Autodesk Inventor part; units mm, degrees
ref_plane "YZ Plane" through (0, 0, 0) normal (1, 0, 0) x (0, 1, 0)
ref_plane "XZ Plane" through (0, 0, 0) normal (0, 1, 0) x (-1, 0, 0)
ref_plane "XY Plane" through (0, 0, 0) normal (0, 0, 1) x (1, 0, 0)
sketch "Эскиз1" plane through (0, 0, 0) normal (0, 1, 0) x (-1, 0, 0)
  line L0 (0, 0) -> (70, 0)
  line L1 (70, 0) -> (70, -90)
  line L2 (70, -90) -> (0, -90)
  line L3 (0, -90) -> (0, 0)
  dimension "d0" = 70
  dimension "d1" = 90
extrude "Выдавливание1" add sketch "Эскиз1" along normal blind 1.5
sketch "Эскиз2" plane through (0, 1.5, 0) normal (0, 1, 0) x (1, 0, 0)
  line L0 (0, 0) -> (0, 90)
  line L1 (0, 0) -> (-7, 0)
  line L2 (-7, 0) -> (-7, 7)
  line L3 (-7, 7) -> (0, 7)
  line L4 (0, 7) -> (0, 0)
  line L5 (-70, 0) -> (0, 0)
  line L6 (-70, 0) -> (-63, 0)
  line L7 (-63, 0) -> (-63, 7)
  line L8 (-63, 7) -> (-70, 7)
  line L9 (-70, 7) -> (-70, 0)
  line L10 (0, 90) -> (-70, 90)
  line L11 (-70, 90) -> (-63, 90)
  line L12 (-63, 90) -> (-63, 83)
  line L13 (-63, 83) -> (-70, 83)
  line L14 (-70, 83) -> (-70, 90)
  line L15 (0, 90) -> (-7, 90)
  line L16 (-7, 90) -> (-7, 83)
  line L17 (-7, 83) -> (0, 83)
  line L18 (0, 83) -> (0, 90)
  point P0 (0, 7)
  point P1 (0, 83)
  point P2 (-63, 0)
  dimension "d4" = 7
  dimension "d5" = 7
  dimension "d6" = 7
  dimension "d7" = 7
  dimension "d8" = 7
  dimension "d9" = 7
  dimension "d10" = 7
  dimension "d11" = 7
extrude "Выдавливание2" add sketch "Эскиз2" along normal blind 5
sketch "Эскиз3" plane through (0, 6.5, 0) normal (0, 1, 0) x (1, 0, 0)
  circle A0 centre (-2.75, 86.25) radius 1.25
  circle A1 centre (-66.25, 86.25) radius 1.25
  circle A2 centre (-66.25, 3.75) radius 1.25
  circle A3 centre (-2.75, 3.75) radius 1.25
  line L0 (-63, 90) -> (-70, 90)
  line L1 (0, 90) -> (-7, 90)
  line L2 (-70, 0) -> (-63, 0)
  line L3 (-7, 0) -> (0, 0)
  line L4 (-70, 90) -> (-70, 83)
  line L5 (0, 7) -> (0, 83)
  line L6 (-70, 7) -> (-70, 0)
  line L7 (0, 0) -> (0, 7)
  dimension "d14" = 2.5
  dimension "d15" = 2.5
  dimension "d16" = 2.5
  dimension "d17" = 2.5
  dimension "d18" = 3.75
  dimension "d19" = 3.75
  dimension "d20" = 3.75
  dimension "d21" = 3.75
  dimension "d22" = 3.75
  dimension "d23" = 2.75
  dimension "d24" = 3.75
  dimension "d25" = 2.75
extrude "Выдавливание3" cut sketch "Эскиз3" against normal blind 5
fillet "Сопряжение1" radius 2 4 edges at (0, 3.25, 0) (0, 3.25, -90) (-70, 3.25, -90) (-70, 3.25, 0)
properties part number "SensorsC_Holder"
Source: CAD feature listing. Evaluate the final solid. Frame: model axes, mm. A direction names the side the tool comes from. Coordinates: 2 decimals unless noted, no trailing zeros. Loops run counter-clockwise (first coordinate to the right, second up) from the corner with the lowest first, then second, coordinate; pieces in that order, holes last. Notation, with made-up numbers: (49, 7) - (98, 7) arc R25 ccw to (98, 34) - close; hole circle Ø9 at (74.5, 50). An arc over 180 degrees is marked (long way). Answer as CSV lines item,"result".
1. Section A-A (y = 4.75). Return loops of the section in (x, z).
Established:
outline,"(-70, -88) arc R2 ccw to (-68, -90) - (-63, -90) - (-63, -83) - (-70, -83) - close; (-70, -7) - (-63, -7) - (-63, 0) - (-68, 0) arc R2 ccw to (-70, -2) - close; (-7, -90) - (-2, -90) arc R2 ccw to (0, -88) - (0, -83) - (-7, -83) - close; (-7, -7) - (0, -7) - (0, -2) arc R2 ccw to (-2, 0) - (-7, 0) - close; hole circle Ø2.5 at (-66.25, -86.25); hole circle Ø2.5 at (-66.25, -3.75); hole circle Ø2.5 at (-2.75, -86.25); hole circle Ø2.5 at (-2.75, -3.75)"
2. Contact query for flat-ended pins moving along their axis: pin 1 (1.5 mm diameter, centred on x = -38, z = -26, fed in from +Y); pin 2 (1.5 mm diameter, centred on x = -10.5, y = 3.5, fed in from +Z). Output: stop coordinate, or through.
Established:
pin 1,"stops at y = 1.5"
pin 2,"passes through"
3. Mould query, pull axis Z, two halves, no side actions, for faces 1 (the cylindrical face through (-65.095, 4.035, -3.271)), 2 (the cylindrical face through (-69.43, 3.2, -89.4)), 3 (the cylindrical face through (-0.6, 3.3, -0.57)), 4 (the flat face through (-7, 4, -3)). Classes: released by +Z, released by -Z, zero draft, split by the parting line, or undercut.
Established:
face 1,"undercut"
face 2,"released by -Z"
face 3,"released by +Z"
face 4,"zero draft"
4. Section C-C (z = -86.25). Return loops of the section in (x, y), then the cut area to 3 significant figures.
Established:
outline,"(-70, 0) - (0, 0) - (0, 6.5) - (-1.5, 6.5) - (-1.5, 1.5) - (-4, 1.5) - (-4, 6.5) - (-7, 6.5) - (-7, 1.5) - (-63, 1.5) - (-63, 6.5) - (-65, 6.5) - (-65, 1.5) - (-67.5, 1.5) - (-67.5, 6.5) - (-70, 6.5) - close"
area,"150 mm2"
5. Section B-B (x = -66.25). Return loops of the section in (y, z).
Established:
outline,"(0, -90) - (6.5, -90) - (6.5, -87.5) - (1.5, -87.5) - (1.5, -85) - (6.5, -85) - (6.5, -83) - (1.5, -83) - (1.5, -7) - (6.5, -7) - (6.5, -5) - (1.5, -5) - (1.5, -2.5) - (6.5, -2.5) - (6.5, 0) - (0, 0) - close"
6. Ray query, line 1 (X direction, y = 5.2, z = -3.75); line 2 (Z direction, x = -66.25, y = 3.3); line 3 (Z direction, x = -64, y = 4). Return the intervals inside material, ascending.
Established:
line 1,"x = -70 to -67.5, -65 to -63, -7 to -4, -1.5 to 0"
line 2,"z = -90 to -87.5, -85 to -83, -7 to -5, -2.5 to 0"
line 3,"z = -90 to -83, -7 to 0"
7. Section D-D (x = -46). Return loops of the section in (y, z).
Established:
outline,"(0, -90) - (1.5, -90) - (1.5, 0) - (0, 0) - close"
8. Reachability of faces 5 (the flat face through (-66, 4, -83)), 6 (the cylindrical face through (-2.173, 4.035, -2.641)), 7 (the flat face through (-7, 4, -87)) from +Z, -Z, +X, -X, +Y, -Y: full face, straight path, thin tool, end or side. Return the list, or none.
Established:
face 5,"+X, -X, +Y"
face 6,"+Y"
face 7,"+Z, -Z, +Y"
